Autodesk Inventor part; units mm, degrees
ref_plane "Work Plane1" through (0, 3.175, 0) normal (0, 1, 0) x (-1, 0, 0)
ref_plane "YZ Plane" through (0, 0, 0) normal (1, 0, 0) x (0, 1, 0)
ref_plane "XY Plane" through (0, 0, 0) normal (0, 0, 1) x (1, 0, 0)
sketch "Sketch1" plane through (0, 0, 0) normal (0, 1, 0) x (-1, 0, 0)
  circle A0 centre (0, 0) radius 68.2625
  dimension "d0" = 136.525
ref_plane "Work Plane1" through (0, 3.175, 0) normal (0, 1, 0) x (-1, 0, 0)
sketch "Sketch2" plane through (0, 3.175, 0) normal (0, 1, 0) x (-1, 0, 0)
  circle A0 centre (0, 0) radius 52.3875
  dimension "d2" = 104.775
loft "Loft1" add profiles "Sketch1", "Sketch2"
sketch "Sketch3" plane through (0, 0, 0) normal (0, -1, 0) x (1, 0, 0)
  circle A0 centre (0, 0) radius 68.2625
extrude "Extrusion1" add sketch "Sketch3" along normal blind 7.62
shell "Shell1" thickness 2.54 removed faces 1 at (13.9501, -7.62, -10.0034)
properties part number "speaker_cover"
Geometry check sheet. Reference: the model listing, model coordinates, mm. A direction names the side the tool comes from. Give positions to 0.01 mm unless a question says otherwise; leave off trailing zeros. Write each loop counter-clockwise with the first axis right and the second up, starting at its lowest first coordinate (ties: lowest second). Pieces come first, ordered by that corner, then holes. Notation, with made-up numbers: (-10, 58.5) - (10, 58.5) arc R27 ccw to (10, 81.5) - close; hole circle Ø8 at (-35, -33.5). An arc over 180 degrees is marked (long way). Put each result on its own line as item: value.
1. Thickness scan on line 1 (X direction, y = -3.3, z = 0); line 2 (Y direction, x = -14.5, z = 18) (3 decimals). Record the ranges inside material, lowest first.
Ans:
line 1: x = -68.26 to -65.72, 65.72 to 68.26
line 2: y = 0.635 to 3.175
2. Go/stop test with flat-tipped pins: pin 1 (5 mm diameter, centred on x = 32, y = 1.5, fed in from +Z); pin 2 (3 mm diameter, centred on x = 44.5, y = -5.5, fed in from +Z); pin 3 (2 mm diameter, centred on x = 12.5, z = -1.5, fed in from -Y) (3 decimals). Record where each tip stops, or that it passes through.
Ans:
pin 1: stops at z = 61.32
pin 2: stops at z = 53.02
pin 3: stops at y = 0.635
3. Set-up check for faces 1 (the flat face through (-36, -7.62, 56)), 2 (the flat face through (1, 0.635, 1)): record each of +Z, -Z, +X, -X, +Y, -Y from which the full face is reachable in a straight line by a thin tool's end or side.
Ans:
face 1: +Z, -Z, +X, -X, -Y
face 2: -Y
4. Sectioned sample at B-B, the plane y = -6. Enter the section's corners in (x, z) (1 decimal).
Ans:
outline: circle Ø136.5 at (0, 0); hole circle Ø131.4 at (0, 0)
5. Sectioned sample at A-A, the plane x = 0. Enter the section's corners in (y, z) (1 decimal), plus the area to 3 significant figures.
Ans:
outline: (-7.6, -68.3) - (0, -68.3) - (3.2, -52.4) - (3.2, 52.4) - (0, 68.3) - (-7.6, 68.3) - (-7.6, 65.7) - (-2.1, 65.7) - (0.6, 52.1) - (0.6, -52.1) - (-2.1, -65.7) - (-7.6, -65.7) - close
area: 375 mm²
6. Draft check along X on faces 3 (the conical face through (11.572, 2.976, 52.111)), 4 (the cylindrical face through (-52.155, -4.812, 39.991)), 5 (the flat face through (1, 3.175, 1)). Enter one of: +X half, -X half, draft (parallel to the pull), parting line (faces both ways), or undercut.
Ans:
face 3: parting line
face 4: undercut
face 5: draft
